Read the model definition and answer for the solid it produces. Units are mm, in the model's axes. A direction names the side the tool comes from. Give positions to 0.01 mm unless a question says otherwise; leave off trailing zeros. Order: outer loops, then holes, each group sorted by start corner. A loop starts at its lowest first (then second) coordinate and runs counter-clockwise, first axis right, second up. Notation, with made-up numbers: M -11.5,82 L 15.5,82 A15 cw 15.5,104 Z; hole C 48.5,-25 d1. An arc over 180 degrees is marked long. One line per item, written item: value. Start each with the question number.
from build123d import *

# Parameters (mm, degrees)
SKETCH_1_R          = 1.75
SKETCH_1_R_2        = 1.5
EXTRUDE_1_DEPTH     = 0.4
SKETCH_2_R          = 1.5
CUT_EXTRUDE_1_DEPTH = 10


with BuildPart() as part:
    # 草图1 → 凸台-拉伸1 (new body)
    with BuildSketch(Plane.XY):
        with BuildLine():
            Line((90, 40.82885301), (-90, 40.82885301))
            ThreePointArc((-90, 40.82885301), (-93.535533906, 39.364386916), (-95, 35.82885301))
            Line((-95, 35.82885301), (-95, -34.17114699))
            ThreePointArc((-95, -34.17114699), (-93.535533906, -37.706680896), (-90, -39.17114699))
            Line((-90, -39.17114699), (90, -39.17114699))
            ThreePointArc((90, -39.17114699), (93.535533906, -37.706680896), (95, -34.17114699))
            Line((95, -34.17114699), (95, 35.82885301))
            ThreePointArc((95, 35.82885301), (93.535533906, 39.364386916), (90, 40.82885301))
        make_face()
        with Locations((-90, -34.17114699)):
            Circle(SKETCH_1_R, mode=Mode.SUBTRACT)
        with BuildLine():
            ThreePointArc((-78.5, -25), (-80, -26.5), (-81.5, -25))
            Line((-81.5, -25), (-81.5, 25))
            ThreePointArc((-81.5, 25), (-80, 26.5), (-78.5, 25))
            Line((-78.5, 25), (-78.5, -25))
        make_face(mode=Mode.SUBTRACT)
        with BuildLine():
            ThreePointArc((-63.5, -25), (-65, -26.5), (-66.5, -25))
            Line((-66.5, -25), (-66.5, 25))
            ThreePointArc((-66.5, 25), (-65, 26.5), (-63.5, 25))
            Line((-63.5, 25), (-63.5, -25))
        make_face(mode=Mode.SUBTRACT)
        with BuildLine():
            ThreePointArc((-43.5, -25), (-45, -26.5), (-46.5, -25))
            Line((-46.5, -25), (-46.5, 25))
            ThreePointArc((-46.5, 25), (-45, 26.5), (-43.5, 25))
            Line((-43.5, 25), (-43.5, -25))
        make_face(mode=Mode.SUBTRACT)
        with BuildLine():
            ThreePointArc((-23.5, -25), (-25, -26.5), (-26.5, -25))
            Line((-26.5, -25), (-26.5, 25))
            ThreePointArc((-26.5, 25), (-25, 26.5), (-23.5, 25))
            Line((-23.5, 25), (-23.5, -25))
        make_face(mode=Mode.SUBTRACT)
        with Locations((0, -35.82885301)):
            Circle(SKETCH_1_R_2, mode=Mode.SUBTRACT)
        with Locations((90, -34.17114699)):
            Circle(SKETCH_1_R, mode=Mode.SUBTRACT)
        with BuildLine():
            Line((-2, 16.362465919), (-2, 13.344643459))
            ThreePointArc((-2, 13.344643459), (-6.746842021, 11.685873172), (-10.55680024, 8.404372537))
            Line((-10.55680024, 8.404372537), (-13.170311155, 9.913283767))
            ThreePointArc((-13.170311155, 9.913283767), (-8.242121859, 14.275773822), (-2, 16.362465919))
        make_face(mode=Mode.SUBTRACT)
        with BuildLine():
            ThreePointArc((-12.55680024, 4.940270922), (-13.493684043, 0), (-12.55680024, -4.940270922))
            Line((-12.55680024, -4.940270922), (-15.170311155, -6.449182152))
            ThreePointArc((-15.170311155, -6.449182152), (-16.484243718, 0), (-15.170311155, 6.449182152))
            Line((-15.170311155, 6.449182152), (-12.55680024, 4.940270922))
        make_face(mode=Mode.SUBTRACT)
        with BuildLine():
            ThreePointArc((-10.55680024, -8.404372537), (-6.746842021, -11.685873172), (-2, -13.344643459))
            Line((-2, -13.344643459), (-2, -16.362465919))
            ThreePointArc((-2, -16.362465919), (-8.242121859, -14.275773822), (-13.170311155, -9.913283767))
            Line((-13.170311155, -9.913283767), (-10.55680024, -8.404372537))
        make_face(mode=Mode.SUBTRACT)
        with BuildLine():
            ThreePointArc((2, -13.344643459), (6.746842021, -11.685873172), (10.55680024, -8.404372537))
            Line((10.55680024, -8.404372537), (13.170311155, -9.913283767))
            ThreePointArc((13.170311155, -9.913283767), (8.242121859, -14.275773822), (2, -16.362465919))
            Line((2, -16.362465919), (2, -13.344643459))
        make_face(mode=Mode.SUBTRACT)
        with BuildLine():
            ThreePointArc((12.55680024, -4.940270922), (13.493684043, 0), (12.55680024, 4.940270922))
            Line((12.55680024, 4.940270922), (15.170311155, 6.449182152))
            ThreePointArc((15.170311155, 6.449182152), (16.484243718, 0), (15.170311155, -6.449182152))
            Line((15.170311155, -6.449182152), (12.55680024, -4.940270922))
        make_face(mode=Mode.SUBTRACT)
        with BuildLine():
            ThreePointArc((10.55680024, 8.404372537), (6.746842021, 11.685873172), (2, 13.344643459))
            Line((2, 13.344643459), (2, 16.362465919))
            ThreePointArc((2, 16.362465919), (8.242121859, 14.275773822), (13.170311155, 9.913283767))
            Line((13.170311155, 9.913283767), (10.55680024, 8.404372537))
        make_face(mode=Mode.SUBTRACT)
        with BuildLine():
            ThreePointArc((26.5, -25), (25, -26.5), (23.5, -25))
            Line((23.5, -25), (23.5, 25))
            ThreePointArc((23.5, 25), (25, 26.5), (26.5, 25))
            Line((26.5, 25), (26.5, -25))
        make_face(mode=Mode.SUBTRACT)
        with BuildLine():
            ThreePointArc((46.5, -25), (45, -26.5), (43.5, -25))
            Line((43.5, -25), (43.5, 25))
            ThreePointArc((43.5, 25), (45, 26.5), (46.5, 25))
            Line((46.5, 25), (46.5, -25))
        make_face(mode=Mode.SUBTRACT)
        with BuildLine():
            ThreePointArc((66.5, -25), (65, -26.5), (63.5, -25))
            Line((63.5, -25), (63.5, 25))
            ThreePointArc((63.5, 25), (65, 26.5), (66.5, 25))
            Line((66.5, 25), (66.5, -25))
        make_face(mode=Mode.SUBTRACT)
        with BuildLine():
            Line((81.5, 25), (81.5, -25))
            ThreePointArc((81.5, -25), (80, -26.5), (78.5, -25))
            Line((78.5, -25), (78.5, 25))
            ThreePointArc((78.5, 25), (80, 26.5), (81.5, 25))
        make_face(mode=Mode.SUBTRACT)
        with Locations((-90, 34.17114699)):
            Circle(SKETCH_1_R, mode=Mode.SUBTRACT)
        with Locations((0, 35.82885301)):
            Circle(SKETCH_1_R_2, mode=Mode.SUBTRACT)
        with Locations((90, 34.17114699)):
            Circle(SKETCH_1_R, mode=Mode.SUBTRACT)
    extrude(amount=EXTRUDE_1_DEPTH)

    # 草图2 → 切除-拉伸1 (cut)
    with BuildSketch(Plane.XY.offset(0.4)):
        Circle(SKETCH_2_R)
    extrude(amount=-CUT_EXTRUDE_1_DEPTH, mode=Mode.SUBTRACT)


solid = part.part
Q1. Find section A-A, the plane x = 4.5. Give the vertices of the cut face in (y, z).
Q2. Each of these flat-tipped pins is pushed along its axis until it touches: pin 1 (8 mm diameter, centred on x = 49.5, y = 31.5, fed in from -Z); pin 2 (2.5 mm diameter, centred on x = 0, y = 35.83, fed in from -Z). Where does it stop, or does it pass through?
Q3. Consider probe 1 along Y at (x, z) = (-90, 0.25); probe 2 along X at (y, z) = (-35.5, 0.15); probe 3 along Y at (x, z) = (-66, 0.3). Determine where each line is inside the solid, lowest interval first.
Q4. A tool of negligible diameter and unlimited length cuts with its end or side. For faces 1 (the cylindrical face through (93.496, -37.745, 0.197)), 2 (the cylindrical face through (6.69, -11.72, 0.2)), from which of +Z, -Z, +X, -X, +Y, -Y can it reach the whole face along a straight path? Write none if from no direction.
Q5. Find section B-B, the plane y = -21.5. State how many separate pieces and enclosed holes the cut face has, then the cut area to 3 significant figures.
Q6. Determine the mould class of faces 3 (the cylindrical face through (-93.5, 39.4, 0.2)), 4 (the cylindrical face through (-8.32, 14.23, 0.2)), 5 (the flat face through (-1.3, 1.4, 0.4)) for opening direction X: released by +X, released by -X, zero draft, split by the parting line, or undercut.
Evaluation:
1. outline: M -39.17,0 L -15.86,0 L -15.86,0.4 L -39.17,0.4 Z; M -12.72,0 L 12.72,0 L 12.72,0.4 L -12.72,0.4 Z; M 15.86,0 L 40.83,0 L 40.83,0.4 L 15.86,0.4 Z
2. pin 1: z = 0
2. pin 2: through
3. probe 1: -39.17 to -35.92, -32.42 to 32.42, 35.92 to 40.83
3. probe 2: -94.82 to -91.14, -88.86 to -1.46, 1.46 to 88.86, 91.14 to 94.82
3. probe 3: -39.17 to -26.12, 26.12 to 40.83
4. face 1: +Z, -Z, +X, -Y
4. face 2: +Z, -Z
5. separate pieces: 9
5. enclosed holes: 0
5. area: 66.4 mm2
6. face 3: released by -X
6. face 4: undercut
6. face 5: zero draft
